Build history of the part. All positions in model axes, mm. A direction names the side the tool comes from. Coordinates: 2 decimals unless noted, no trailing zeros. Loops run counter-clockwise (first coordinate to the right, second up) from the corner with the lowest first, then second, coordinate; pieces in that order, holes last.
(1) Slice it at C-C (y = -9.5). Give the cut face in (x, z).
(2) Slice it at A-A (y = -14.5). Give the cut face in (x, z).
(3) Slice it at B-B (x = 7.5). Give the cut face in (y, z).
(4) Tool access for faces 1 (the face through (25, 0, 27)), 2 (the face through (38.1, -6, 35)), 3 (the face through (22, -25.4, 63)), 4 (the face through (12.7, -6, 35)): list every direction of +Z, -Z, +X, -X, +Y, -Y with a clear straight run to the whole face (end or side of a thin tool).
(5) Two-plate mould, pull along Y, no slides. Class faces 5 (the face through (39.46, -37.8, 3.22)), 6 (the face through (10.213, -31.885, 3.219)), 7 (the face through (25, -28, 6.35)), 8 (the face through (25, -12.7, 26)): pulls with the +Y half, pulls with the -Y half, needs draft (parallel to the pull), parting line crosses it, or undercut.
(6) Wall check: L1, parallel to Z at x = 25.4, y = -16.25; L2, parallel to X at y = -9.75, z = 57.15; L3, parallel to Y at x = 32, z = 56.5. Give the ranges that are in metal, low to high.
(7) Flat gauge pins, fed straight in: P1, Ø12, axis at x = 6, z = 14.5, coming from the +Y side; P2, Ø1.5, axis at x = 41, y = -17, coming from the +Z side; P3, Ø10, axis at y = -3.5, z = 41, coming from the +X side; P4, Ø10, axis at x = 15.5, z = 28, coming from the -Y side. Where does each tip first touch, or does it go through?
from build123d import *

# Parameters (mm, degrees)
F1_DEPTH = 50.8
F3_DEPTH = 12.7
F5_R     = 3.175
F6_DEPTH = 6.351
F8_DEPTH = 6.351
F9_DEPTH = 44.451


with BuildPart() as f1:
    # F0 (on Right) → F1 (new body)
    with BuildSketch(Plane.YZ):
        Polygon((-44.45, 0), (0, 0), (0, 69.85), (-12.7, 69.85), (-12.7, 6.35), (-44.45, 6.35), align=None)
    extrude(amount=F1_DEPTH)

    # F2 (on face) → F3 (join)
    with BuildSketch(Plane.XZ.offset(12.7)):
        with BuildLine():
            ThreePointArc((38.1, 57.15), (34.3802561211, 66.1302561211), (25.4, 69.85))
            ThreePointArc((25.4, 69.85), (16.4197438789, 48.1697438789), (38.1, 57.15))
        make_face()
        with BuildLine():
            ThreePointArc((31.75, 57.15), (20.9098719395, 52.6598719395), (25.4, 63.5))
            ThreePointArc((25.4, 63.5), (29.8901280605, 61.6401280605), (31.75, 57.15))
        make_face(mode=Mode.SUBTRACT)
    extrude(amount=F3_DEPTH)

    # F5 (on face) → F6 (cut, through all)
    with BuildSketch(Plane.XY.offset(6.35)):
        with BuildLine():
            ThreePointArc((12.7, -34.9846648967), (9.525, -31.8096648967), (6.35, -34.9846648967))
            ThreePointArc((6.35, -34.9846648967), (9.525, -38.1596648967), (12.7, -34.9846648967))
        make_face()
        with Locations((37.9935720786, -34.9846648967)):
            Circle(F5_R)
    extrude(amount=-F6_DEPTH, mode=Mode.SUBTRACT)

    # F7 (on face) → F8 (cut, through all)
    with BuildSketch(Plane.XY.offset(6.35)):
        with BuildLine():
            Line((9.525, -38.1596648967), (9.525, -34.9846648967))
            Line((9.525, -34.9846648967), (6.35, -34.9846648967))
            ThreePointArc((6.35, -34.9846648967), (7.2799359697, -37.229728927), (9.525, -38.1596648967))
        make_face()
    extrude(amount=-F8_DEPTH, mode=Mode.SUBTRACT)

    # F4 (on face) → F9 (cut, through all)
    with BuildSketch(Plane(origin=(0, 0, 0), x_dir=(-1, 0, 0), z_dir=(0, 1, 0))):
        with BuildLine():
            ThreePointArc((-50.8, 6.35), (-43.4796733765, 7.5843467529), (-38.1, 12.7))
            Line((-38.1, 12.7), (-50.8, 12.7))
            Line((-50.8, 12.7), (-50.8, 6.35))
        make_face()
        with BuildLine():
            ThreePointArc((-38.1, 57.15), (-34.3802561211, 66.1302561211), (-25.4, 69.85))
            Line((-25.4, 69.85), (-50.8, 69.85))
            Line((-50.8, 69.85), (-50.8, 12.7))
            Line((-50.8, 12.7), (-38.1, 12.7))
            Line((-38.1, 12.7), (-38.1, 57.15))
        make_face()
        with BuildLine():
            Line((0, 69.85), (-25.4, 69.85))
            ThreePointArc((-25.4, 69.85), (-16.4197438789, 66.1302561211), (-12.7, 57.15))
            Line((-12.7, 57.15), (-12.7, 12.7))
            ThreePointArc((-12.7, 12.7), (-7.3203266235, 7.5843467529), (0, 6.35))
            Line((0, 6.35), (0, 69.85))
        make_face()
        with BuildLine():
            ThreePointArc((-19.05, 57.15), (-20.9098719395, 61.6401280605), (-25.4, 63.5))
            ThreePointArc((-25.4, 63.5), (-29.8901280605, 52.6598719395), (-19.05, 57.15))
        make_face()
    extrude(amount=-F9_DEPTH, mode=Mode.SUBTRACT)


solid = f1.part
Response values:
1. outline: (0, 0) - (50.8, 0) - (50.8, 6.35) arc R12.7 cw to (38.1, 12.7) - (38.1, 57.15) arc R12.7 ccw to (12.7, 57.15) - (12.7, 12.7) arc R12.7 cw to (0, 6.35) - close; hole circle Ø12.7 at (25.4, 57.15)
2. outline: (0, 0) - (50.8, 0) - (50.8, 6.35) arc R12.7 cw to (47.52, 6.35) - (3.28, 6.35) arc R12.7 cw to (0, 6.35) - close; circle Ø25.4 at (25.4, 57.15); hole circle Ø12.7 at (25.4, 57.15)
3. outline: (-44.45, 0) - (-37.43, 0) - (-37.43, 6.35) - (-44.45, 6.35) - close; (-32.54, 0) - (0, 0) - (0, 7.68) - (-12.7, 7.68) - (-12.7, 6.35) - (-32.54, 6.35) - close
4. face 1: +Z, -Z, +X, -X, +Y
4. face 2: +Z, +X, +Y, -Y
4. face 3: +Z, +X, -X, -Y
4. face 4: +Z, -X, +Y, -Y
5. face 5: undercut
5. face 6: undercut
5. face 7: needs draft
5. face 8: pulls with the -Y half
6. L1: z = 0 to 6.35, 44.45 to 50.8, 63.5 to 69.85
6. L2: x = 12.7 to 19.05, 31.75 to 38.1
6. L3: y = -25.4 to 0
7. P1: passes through
7. P2: stops at z = 6.35
7. P3: stops at x = 38.1
7. P4: stops at y = -12.7
